Geometry check sheet. Reference: drawing and pictorial views, mm from the part's lowest x, y, z. A direction names the side the tool comes from. Coordinates: 2 decimals unless noted, no trailing zeros. Write each loop counter-clockwise with the first axis right and the second up, starting at its lowest first coordinate (ties: lowest second). Pieces come first, ordered by that corner, then holes. Notation, with made-up numbers: (-26.5, -39) -> (16.5, -39) arc R23 ccw to (16.5, -18) -> close; hole circle Ø8 at (23, 19). An arc over 180 degrees is marked (long way). Put each result on its own line as item: value.
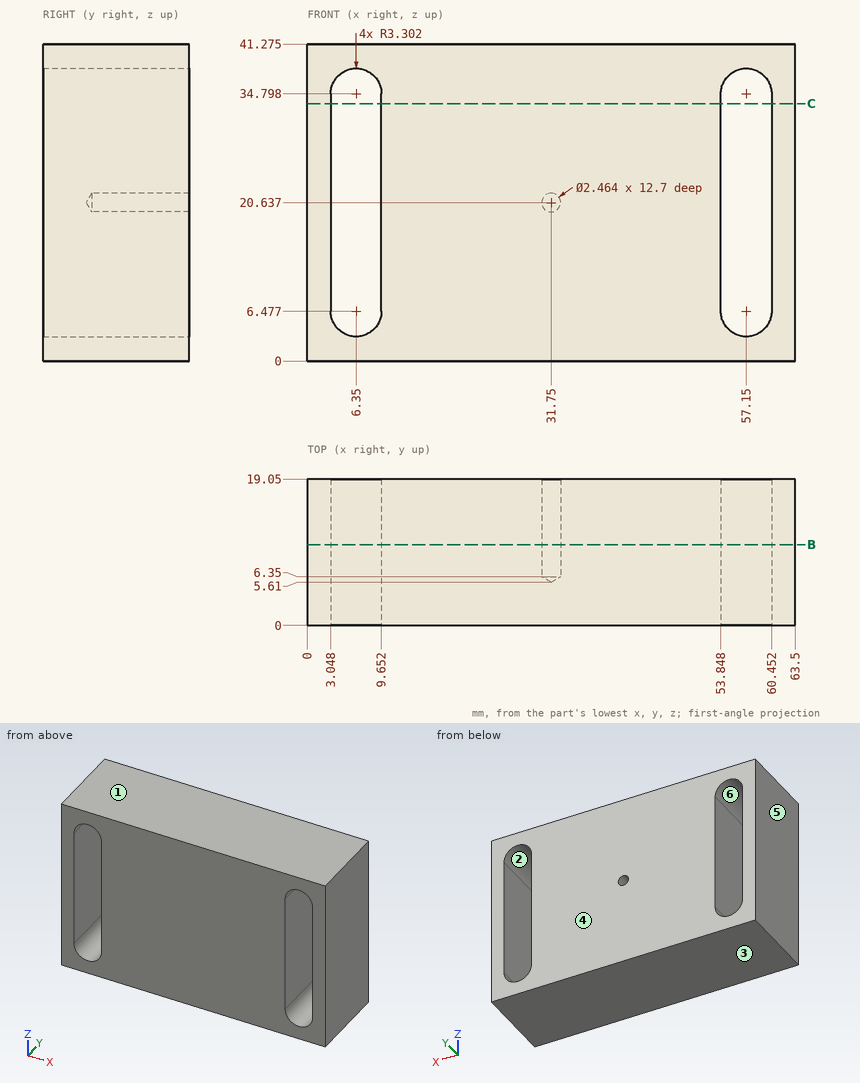
Q1. Cross-section at C-C (z = 33.5). Record the cut outline in (x, y).
Recorded:
outline: (0, 0) -> (3.05, 0) -> (3.05, 19.05) -> (0, 19.05) -> close; (9.65, 0) -> (53.85, 0) -> (53.85, 19.05) -> (9.65, 19.05) -> close; (60.45, 0) -> (63.5, 0) -> (63.5, 19.05) -> (60.45, 19.05) -> close
Q2. Tool access check on the marked faces 5 and 6. Record the directions out of +Z, -Z, +X, -X, +Y, -Y that give a thin tool (end or side, any length) a straight path to the whole face; none if there is none.
Recorded:
face 5: +Z, -Z, -X, +Y, -Y
face 6: +Y, -Y
Q3. Mould release check, pull along Z, two halves, no side actions. Record for the marked faces 1, 2, 3 and 4: released by +Z, released by -Z, zero draft, split by the parting line, or undercut.
Recorded:
face 1: released by +Z
face 2: undercut
face 3: released by -Z
face 4: zero draft
Q4. Cross-section at B-B (y = 10.5). State how many separate pieces and enclosed holes the cut face has, plus the area to 3 significant figures.
Recorded:
separate pieces: 1
enclosed holes: 3
area: 2,170 mm2
Q5. Material ranges on line 1 along X through (y, z) = (5.5, 29); line 2 along X through (y, z) = (11.5, 21); line 3 along X through (y, z) = (17.25, 3.5) (1 decimal), recorded low to high.
Recorded:
line 1: x = 0 to 3.05, 9.65 to 53.85, 60.45 to 63.5
line 2: x = 0 to 3.05, 9.65 to 30.57, 32.93 to 53.85, 60.45 to 63.5
line 3: x = 0 to 4.9, 7.8 to 55.7, 58.6 to 63.5
